For this review, take the finished solid that the model builds, in its own axes (mm). Coordinates: 2 decimals unless noted, no trailing zeros. Order: outer loops, then holes, each group sorted by start corner. A loop starts at its lowest first (then second) coordinate and runs counter-clockwise, first axis right, second up. Notation, with made-up numbers: (6, 5.25) -> (24, 5.25) arc R22 cw to (24, 38.25) -> close; hole circle Ø10 at (-20, 40.5). An arc over 180 degrees is marked (long way). Return JSON: item names as keys, results as strings. Group by question number.
Item 1: For line 1 along Y through (x, z) = (0, 7.75); line 2 along Y through (x, z) = (0, 3); line 3 along Z through (x, y) = (-3.5, 3.25), list the stretches that pass through material, from the lowest coordinate up.
Item 2: Take a section at C-C (z = 2). Write out the cut boundary in (x, y).
Item 3: Take a section at D-D (x = -1.25). Write out the cut boundary in (y, z).
Item 4: Take a section at B-B (x = 0). Write out the cut boundary in (y, z), then the cut area to 3 significant figures.
Item 5: Insertion check: pin 1 (2 mm diameter, centred on x = 2, z = 12, fed in from +Y); pin 2 (2 mm diameter, centred on x = -2, y = 2, fed in from +Z). Each pin has a flat end and moves straight along its axis. Give the tip position at first contact, or say it passes through.
Item 6: Draft analysis for pull direction X (two halves, no side actions). For faces 1 (the cylindrical face through (0, 0, 9)), 2 (the cylindrical face through (0, 4, 2)), 3 (the flat face through (-4, -8, 7)), 4 (the flat face through (0, -19.895, 7)), state which applies: +X half, -X half, draft (parallel to the pull), parting line (faces both ways), or undercut.
Item 7: Take a section at A-A (y = -10). Write out the cut boundary in (x, z).
Autodesk Inventor part; units mm, degrees
ref_plane "YZ Plane" through (0, 0, 0) normal (1, 0, 0) x (0, 1, 0)
ref_plane "XZ Plane" through (0, 0, 0) normal (0, 1, 0) x (-1, 0, 0)
ref_plane "XY Plane" through (0, 0, 0) normal (0, 0, 1) x (1, 0, 0)
sketch "Sketch1" plane through (0, 0, 0) normal (0, 0, 1) x (1, 0, 0)
  arc A0 (-4, 0.1053) -> (4, 0.1053) centre (0, 76) ccw
  line L0 (4, 0.1053) -> (4, -19.8947)
  line L1 (4, -19.8947) -> (-4, -19.8947)
  line L2 (-4, -19.8947) -> (-4, 0.1053)
  arc A1 (-4, 4.1112) -> (4, 4.1112) centre (0, 76) ccw
  line L3 (4, 0.1053) -> (4, 4.1112)
  line L4 (-4, 0.1053) -> (-4, 4.1112)
  point P0 (0, 0)
  point P1 (0, -19.8947)
  point P2 (0, 0)
  dimension "d0" = 76
  dimension "d1" = 4
  dimension "d2" = 8
  dimension "d3" = 20
extrude "Extrusion1" add sketch "Sketch1" along normal blind 14 contours A0 L0 L1 L2
extrude "Extrusion2" add sketch "Sketch1" along normal blind 4 contours L4 A1 L3 A0
sketch "Sketch2" plane through (0, 0, 14) normal (0, 0, 1) x (1, 0, 0)
  circle A0 centre (0, -10) radius 1.7
  arc A1 (-4, 0.1053) -> (4, 0.1053) centre (0, 76) ccw
  point P0 (0, 0)
  point P1 (0, 0)
  dimension "d11" = 0
  dimension "d8" = 3.4
  dimension "d9" = 10
extrude "Extrusion3" cut sketch "Sketch2" against normal through all
properties part number "holder"
Findings below:
{
 "1": {"line 1": "y = -19.89 to -11.7, -8.3 to 0", "line 2": "y = -19.89 to -11.7, -8.3 to 4", "line 3": "z = 0 to 4"},
 "2": {"outline": "(-4, -19.89) -> (4, -19.89) -> (4, 4.11) arc R72 cw to (-4, 4.11) -> close; hole circle Ø3.4 at (0, -10)"},
 "3": {"outline": "(-19.89, 0) -> (-11.15, 0) -> (-11.15, 14) -> (-19.89, 14) -> close; (-8.85, 0) -> (4.01, 0) -> (4.01, 4) -> (0.01, 4) -> (0.01, 14) -> (-8.85, 14) -> close"},
 "4": {"outline": "(-19.89, 0) -> (-11.7, 0) -> (-11.7, 14) -> (-19.89, 14) -> close; (-8.3, 0) -> (4, 0) -> (4, 4) -> (0, 4) -> (0, 14) -> (-8.3, 14) -> close", "area": "247 mm2"},
 "5": {"pin 1": "stops at y = 0.06", "pin 2": "stops at z = 4"},
 "6": {"face 1": "undercut", "face 2": "undercut", "face 3": "-X half", "face 4": "draft"},
 "7": {"outline": "(-4, 0) -> (-1.7, 0) -> (-1.7, 14) -> (-4, 14) -> close; (1.7, 0) -> (4, 0) -> (4, 14) -> (1.7, 14) -> close"}
}
